```python
from build123d import *

# Parameters (mm, degrees)
BOSS_EXTRUDE1_DEPTH            = 3
M6_CLEARANCE_HOLE1_D           = 6.6
M6_CLEARANCE_HOLE1_DEPTH       = 12
M6_CLEARANCE_HOLE1_CSINK_D     = 6.65
M6_CLEARANCE_HOLE1_CSINK_ANGLE = 90
M6_CLEARANCE_HOLE1_TIP         = 1.982840043


with BuildPart() as part:
    # Sketch1 → Boss-Extrude1 (new body)
    with BuildSketch(Plane(origin=(0, 0, 0), x_dir=(1, 0, 0), z_dir=(0, 1, 0))):
        Polygon((6.35, 6.35), (82.7, 82.7), (82.7, 565.66051224), (-82.7, 565.66051224), (-82.7, 82.7), (-6.35, 6.35), (-6.35, 30.27243444), (6.35, 30.27243444), align=None)
    extrude(amount=-BOSS_EXTRUDE1_DEPTH)

    # M6 Clearance Hole1
    with Locations(Plane(origin=(-73.056682922, 0, -550.13126836), x_dir=(0, 0, 1), z_dir=(0, 1, 0))):
        with Locations((0, 0), (0, 146.113365844), (225.95101224, 0), (225.95101224, 146.113365844), (467.43126836, 146.113365844), (467.43126836, 0), (497.696436729, 47.041768684), (497.696436729, 99.07159716)):
            CounterSinkHole(M6_CLEARANCE_HOLE1_D / 2, M6_CLEARANCE_HOLE1_CSINK_D / 2, depth=M6_CLEARANCE_HOLE1_DEPTH, counter_sink_angle=M6_CLEARANCE_HOLE1_CSINK_ANGLE)
            with Locations((0, 0, -(M6_CLEARANCE_HOLE1_DEPTH + M6_CLEARANCE_HOLE1_TIP / 2))):  # 118° drill point
                Cone(0, M6_CLEARANCE_HOLE1_D / 2, M6_CLEARANCE_HOLE1_TIP, mode=Mode.SUBTRACT)


solid = part.part
```
Model file for the job. Use its own axes, mm. Give positions to 0.01 mm unless a question says otherwise; leave off trailing zeros. Write each loop counter-clockwise with the first axis right and the second up, starting at its lowest first coordinate (ties: lowest second). Pieces come first, ordered by that corner, then holes. Notation, with made-up numbers: (16, 26.25) - (68, 26.25) arc R20 cw to (68, 53.25) - close; hole circle Ø6 at (-6.5, 82). An arc over 180 degrees is marked (long way). One line per question, with ' | ' between items. Start each with the question number.
(1) Wall check: line 1 along X through (y, z) = (-1.6, -82.7); line 2 along Z through (x, y) = (75.5, -2.85); line 3 along Z through (x, y) = (-23, -1). Give the ranges that are in metal, low to high. Write a range as from..to.
(2) Slice it at B-B on x = -46. Write the cut outline in (y, z), plus the area to 3 significant figures.
(3) Slice it at A-A on y = -1.3. Give the number of separate pieces and of enclosed holes in the cut face, plus the area to 3 significant figures.
(4) Slice it at C-C on x = 48. Write the cut outline in (y, z).
(5) Pin check, flat tips, straight feed: P1, Ø4, axis at x = 73.06, z = -550.13, coming from the +Y side; P2, Ø1, axis at x = -46, y = -2.5, coming from the +Z side; P3, Ø1.5, axis at y = -2, z = -23, coming from the +X side; P4, Ø0.9, axis at y = -2, z = -13.5, coming from the -X side. Stop position of each tip, or through.
Results below:
1) line 1: -82.7..-76.36, -69.76..69.76, 76.36..82.7 | line 2: -565.66..-552.35, -547.91..-326.4, -321.96..-84.92, -80.48..-75.5 | line 3: -565.66..-53.78, -51.09..-23
2) outline: (-3, -565.66) - (0, -565.66) - (0, -46) - (-3, -46) - close | area: 1,560 mm^2
3) separate pieces: 1 | enclosed holes: 8 | area: 86,100 mm^2
4) outline: (-3, -565.66) - (0, -565.66) - (0, -48) - (-3, -48) - close
5) P1: through | P2: z = -45.5 | P3: x = 23.75 | P4: x = -13.95
